from build123d import *

# Parameters (mm, degrees)
F0_R     = 45
F1_DEPTH = 110
F2_T     = -3
F3_R     = 2
F4_R     = 2
F5_R     = 2
F7_DEPTH = 1


# Not quite as in the source:
# - a fillet or chamfer that OpenCascade refuses, or shapes differently, is made with other operations: its cross-section is extruded or revolved along the edge and cut away or added


with BuildPart() as f1:
    # F0 (on Top) → F1 (new body)
    with BuildSketch(Plane.XY):
        Circle(F0_R)
    extrude(amount=F1_DEPTH)

    # F2
    f2_openings = [f1.faces().sort_by_distance(p)[0] for p in [
        (0, 0, 110),
    ]]
    offset(amount=F2_T, openings=f2_openings)

    # F3
    f3_edges = [f1.edges().sort_by_distance(p)[0] for p in [
        (-42, 0, 3),
    ]]
    fillet(f3_edges, radius=F3_R)

    # F4
    f4_edges = [f1.edges().sort_by_distance(p)[0] for p in [
        (-45, 0, 0),
    ]]
    fillet(f4_edges, radius=F4_R)

    # F5
    f5_edges = [f1.edges().sort_by_distance(p)[0] for p in [
        (-45, 0, 110),
    ]]
    fillet(f5_edges, radius=F5_R)

    # F6: fillet of radius 2 on 1 edges, made by hand

    # F6_s1 → F6_t2 (revolve, cut)
    with BuildSketch(Plane.XZ):
        with BuildLine():
            ThreePointArc((42.9997999035, 110.0003463544), (42.2675927526, 109.2678330874), (41.9996, 108.2673917434))
            Line((41.9996, 108.2673917434), (41.7994634315, 108.2673917434))
            ThreePointArc((41.7994634315, 108.2673917434), (41.7998634315, 109.1336958717), (41.7998634315, 110))
            Line((41.7998634315, 110), (42, 110.2001365685))
            ThreePointArc((42, 110.2001365685), (42.4998999517, 110.2001365685), (42.8996833253, 110.1736418155))
            Line((42.8996833253, 110.1736418155), (42.9997999035, 110.0003463544))
        make_face()
    revolve(axis=Axis((0, 0, 110), (0, 0, 1)), mode=Mode.SUBTRACT)

    # F7 (cut): a face of the model
    f7_faces = [f1.faces().sort_by_distance(p)[0] for p in [
        (0, 0, 0),
    ]]
    extrude(f7_faces, amount=-F7_DEPTH, mode=Mode.SUBTRACT)

    # F8: fillet of radius 1 on 1 edges, made by hand

    # F8_s1 → F8_t2 (revolve, cut)
    with BuildSketch(Plane.XZ):
        with BuildLine():
            ThreePointArc((44.7320508076, 1), (43.8660254038, 0.5), (43, 1))
            Line((43, 1), (43, 0))
            ThreePointArc((43, 0), (44, 0.2679491924), (44.7320508076, 1))
        make_face()
    revolve(axis=Axis((0, 0, 0), (0, 0, 1)), mode=Mode.SUBTRACT)


solid = f1.part
The listing builds one solid part. Answer for the finished solid, in the listing's coordinates (mm). A direction names the side the tool comes from. Round coordinates to 2 decimals unless told otherwise and drop trailing zeros. Order: outer loops, then holes, each group sorted by start corner. A loop starts at its lowest first (then second) coordinate and runs counter-clockwise, first axis right, second up. Notation, with made-up numbers: M -21,14.5 L 11,14.5 A14 cw 11,25.5 Z; hole C 17.5,68.25 d9. An arc over 180 degrees is marked long. Answer in a Markdown table with one row per item. Add a question column.
1) Flat-ended cylindrical pins translate along their axes: pin 1 Ø12 at (x, y) = (4.5, 28) entering from -Z; pin 2 Ø4 at (x, y) = (-9.5, 8.5) entering from +Z; pin 3 Ø10 at (x, z) = (-16.5, 44.5) entering from +Y. Find the tip coordinate at first contact, or state that the pin passes through.
2) Determine the mould class of faces 1 (the face through (-1, 1, 3)), 2 (the face through (20.765, -39.923, 54.258)) for opening direction Y: pulls with the +Y half, pulls with the -Y half, needs draft (parallel to the pull), parting line crosses it, or undercut.
3) Which of the six approach directions +Z, -Z, +X, -X, +Y, -Y give full straight-line access (tool end or side, diameter ignored) to faces 3 (the face through (-1, 1, 1)), 4 (the face through (40.06, 12.62, 55.93))?
4) Consider line 1 along Y through (x, z) = (0, 70); line 2 along Z through (x, y) = (-7, 23); line 3 along Y through (x, z) = (14.5, 16). Determine where each line is inside the solid, lowest interval first. Write a range as from..to.
5) The part is cut by section C-C on z = 12.5. Determine the outline of the cut face in (x, y), plus the area to 3 significant figures.
Findings below:
| question | item | result |
|---|---|---|
| 1 | pin 1 | stops at z = 1 |
| 1 | pin 2 | stops at z = 3 |
| 1 | pin 3 | stops at y = 43.51 |
| 2 | face 1 | undercut |
| 2 | face 2 | parting line crosses it |
| 3 | face 3 | -Z |
| 3 | face 4 | +Z |
| 4 | line 1 | y = -45..-42, 42..45 |
| 4 | line 2 | z = 1..3 |
| 4 | line 3 | y = -42.6..-39.42, 39.42..42.6 |
| 5 | outline | C 0,0 d90; hole C 0,0 d84 |
| 5 | area | 820 mm² |
